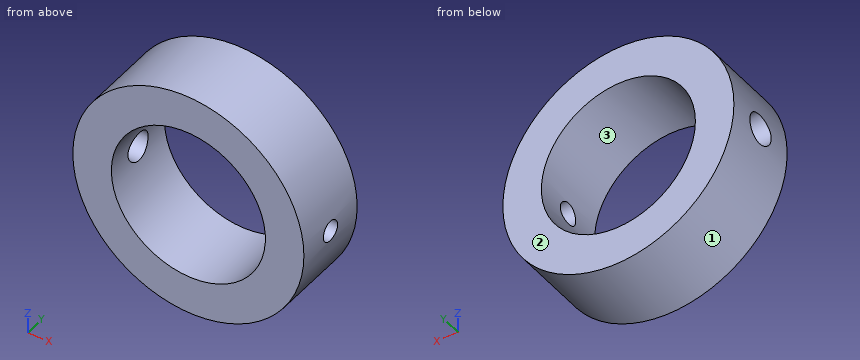
Autodesk Inventor part; units mm, degrees
ref_plane "YZ Plane" through (0, 0, 0) normal (1, 0, 0) x (0, 1, 0)
ref_plane "XZ Plane" through (0, 0, 0) normal (0, 1, 0) x (-1, 0, 0)
ref_plane "XY Plane" through (0, 0, 0) normal (0, 0, 1) x (1, 0, 0)
sketch "Sketch1" plane through (0, 0, 0) normal (0, 1, 0) x (-1, 0, 0)
  circle A0 centre (0, 0) radius 22.5
  circle A1 centre (0, 0) radius 15
  dimension "d0" = 45
  dimension "d1" = 30
extrude "Extrusion1" add sketch "Sketch1" along normal mid plane 15
sketch "Sketch2" plane through (0, 0, 0) normal (0, 0, 1) x (1, 0, 0)
  line L0 (-22.5, -7.5) -> (-22.5, 7.5)
  line L1 (-22.5, 0) -> (22.5, 0)
  line L2 (22.5, -7.5) -> (22.5, 7.5)
  line L3 (-22.5, 0) -> (-22.5, 3)
  line L4 (22.5, 0) -> (22.5, 2)
  line L5 (22.5, 2) -> (-22.5, 3)
  point P0 (0, 0)
  dimension "d4" = 3
  dimension "d5" = 2
revolve "Revolution1" cut sketch "Sketch2" angle 360 about axis through (-22.5, 0, 0) along (1, 0, 0)
properties part number "taper pin"
Part model, mm, in its own coordinate system. Face numbers are marked on the shaded views. Give positions to 0.01 mm unless a question says otherwise; leave off trailing zeros. Order: outer loops, then holes, each group sorted by start corner. A loop starts at its lowest first (then second) coordinate and runs counter-clockwise, first axis right, second up. Notation, with made-up numbers: (-28, -7) -> (14, -7) arc R33 cw to (14, 26) -> close; hole circle Ø8 at (35.5, 40.25). An arc over 180 degrees is marked (long way). Use one line per item in the form item = value.
(1) Saw through at C-C (y = 0). Write the cut outline in (x, z), then the cut area to 3 significant figures.
Solution:
outline = (-22.3, -3) arc R22.5 ccw to (22.41, -2) -> (14.84, -2.17) arc R15 cw to (-14.73, -2.83) -> close; (-22.3, 3) -> (-14.73, 2.83) arc R15 cw to (14.84, 2.17) -> (22.41, 2) arc R22.5 ccw to start
area = 808 mm²
(2) Saw through at A-A (x = -18). Write the cut outline in (y, z).
Solution:
outline = (-7.5, -13.5) -> (7.5, -13.5) -> (7.5, 13.5) -> (-7.5, 13.5) -> close; hole circle Ø5.8 at (0, 0)
(3) Saw through at B-B (x = 0). Write the cut outline in (y, z), then the cut area to 3 significant figures.
Solution:
outline = (-7.5, -22.5) -> (7.5, -22.5) -> (7.5, -15) -> (-7.5, -15) -> close; (-7.5, 15) -> (7.5, 15) -> (7.5, 22.5) -> (-7.5, 22.5) -> close
area = 225 mm²
(4) Drill centre lines: line 1 (X direction, y = -6, z = 0); line 2 (X direction, y = 2.5, z = -6.5). Where is each one in solid material? Low to high. Write a range as from..to.
Solution:
line_1 = -22.5..-15, 15..22.5
line_2 = -21.54..-13.52, 13.52..21.54
(5) Flat gauge pins, fed straight in: P1, Ø8, axis at y = 4, z = -14.5, coming from the -X side; P2, Ø1.5, axis at x = 12.5, y = 4, coming from the +Z side; P3, Ø18, axis at x = 0, z = 0, coming from the -Y side; P4, Ø5, axis at x = 15.5, y = -1, coming from the -Z side. Where does each tip first touch, or does it go through?
Solution:
P1 = -19.9
P2 = 19.19
P3 = through
P4 = -18.36
(6) Pull direction X, two halves, no side cores. Call the marked faces 1, 2 and 3: +X half, -X half, draft (parallel to the pull), parting line (faces both ways), or undercut.
Solution:
face_1 = parting line
face_2 = draft
face_3 = undercut
(7) Saw through at D-D (z = 0). Write the cut outline in (x, y), then the cut area to 3 significant figures.
Solution:
outline = (-22.5, -7.5) -> (-15, -7.5) -> (-15, -2.83) -> (-22.5, -3) -> close; (-22.5, 3) -> (-15, 2.83) -> (-15, 7.5) -> (-22.5, 7.5) -> close; (15, -7.5) -> (22.5, -7.5) -> (22.5, -2) -> (15, -2.17) -> close; (15, 2.17) -> (22.5, 2) -> (22.5, 7.5) -> (15, 7.5) -> close
area = 150 mm²
